```python
from build123d import *

# Parameters (mm, degrees)
SKETCH_1_W          = 47
SKETCH_1_H          = 47
EXTRUDE_1_DEPTH     = 17
SKETCH_2_R          = 2.1
CUT_EXTRUDE_1_DEPTH = 69.607579756
SKETCH_3_W          = 34.6
SKETCH_3_H          = 34.6
CUT_EXTRUDE_2_DEPTH = 14.25
FILLET_1_R          = 2
FILLET_2_R          = 1.5
CHAMFER_1_SIZE      = 1.5
FILLET_3_R          = 1.5


with BuildPart() as part:
    # Эскиз1 → Бобышка-Вытянуть1 (new body)
    with BuildSketch(Plane(origin=(0, 0, 0), x_dir=(1, 0, 0), z_dir=(0, 1, 0))):
        with Locations((-23.5, 23.5)):
            Rectangle(SKETCH_1_W, SKETCH_1_H)
    extrude(amount=EXTRUDE_1_DEPTH)

    # Эскиз2 → Вырез-Вытянуть1 (cut, through all)
    with BuildSketch(Plane.XZ):
        with Locations(Location((-43.5, -3.5, 0), (0, 0, 270))):
            Circle(SKETCH_2_R)
        with Locations(Location((-3.5, -3.5, 0), (0, 0, 90))):
            Circle(SKETCH_2_R)
        with Locations(Location((-3.5, -43.5, 0), (0, 0, 270))):
            Circle(SKETCH_2_R)
        with Locations(Location((-43.5, -43.5, 0), (0, 0, 90))):
            Circle(SKETCH_2_R)
    extrude(amount=-CUT_EXTRUDE_1_DEPTH, mode=Mode.SUBTRACT)

    # Эскиз3 → Вырез-Вытянуть2 (cut)
    with BuildSketch(Plane.XZ):
        with Locations((-23.5, -23.5)):
            Rectangle(SKETCH_3_W, SKETCH_3_H)
    extrude(amount=-CUT_EXTRUDE_2_DEPTH, mode=Mode.SUBTRACT)

    # Скругление1
    fillet_1_edges = [part.edges().sort_by_distance(p)[0] for p in [
        (0, 8.5, 0),
        (-47, 8.5, 0),
        (-47, 8.5, -47),
        (0, 8.5, -47),
    ]]
    fillet(fillet_1_edges, radius=FILLET_1_R)

    # Скругление2
    fillet_2_edges = [part.edges().sort_by_distance(p)[0] for p in [
        (-40.8, 14.25, -23.5),
        (-23.5, 14.25, -6.2),
        (-6.2, 14.25, -23.5),
        (-23.5, 14.25, -40.8),
    ]]
    fillet(fillet_2_edges, radius=FILLET_2_R)

    # Фаска1
    # the kernel refuses this chamfer: 1.5 mm, written as the material it takes off along each edge
    with BuildSketch(Plane(origin=(-43.5, 17, -43.5), x_dir=(0, 0, 1), z_dir=(1, 0, 0))) as chamfer_1_piece_1:
        Polygon((2.1, CHAMFER_1_SIZE), (2.1 + CHAMFER_1_SIZE, 0), (2.1, 0), align=None)
    revolve(axis=Axis((-43.5, 17, -43.5), (0, -1, 0)), mode=Mode.SUBTRACT)
    with BuildSketch(Plane(origin=(-3.5, 17, -43.5), x_dir=(0, 0, -1), z_dir=(-1, 0, 0))) as chamfer_1_piece_2:
        Polygon((2.1, CHAMFER_1_SIZE), (2.1 + CHAMFER_1_SIZE, 0), (2.1, 0), align=None)
    revolve(axis=Axis((-3.5, 17, -43.5), (0, -1, 0)), mode=Mode.SUBTRACT)
    with BuildSketch(Plane(origin=(-3.5, 17, -3.5), x_dir=(0, 0, 1), z_dir=(1, 0, 0))) as chamfer_1_piece_3:
        Polygon((2.1, CHAMFER_1_SIZE), (2.1 + CHAMFER_1_SIZE, 0), (2.1, 0), align=None)
    revolve(axis=Axis((-3.5, 17, -3.5), (0, -1, 0)), mode=Mode.SUBTRACT)
    with BuildSketch(Plane(origin=(-43.5, 17, -3.5), x_dir=(0, 0, -1), z_dir=(-1, 0, 0))) as chamfer_1_piece_4:
        Polygon((2.1, CHAMFER_1_SIZE), (2.1 + CHAMFER_1_SIZE, 0), (2.1, 0), align=None)
    revolve(axis=Axis((-43.5, 17, -3.5), (0, -1, 0)), mode=Mode.SUBTRACT)

    # Скругление3
    # the kernel refuses this fillet: 1.5 mm, written as the material it adds along each edge
    with BuildSketch(Plane(origin=(-39.3, 12.75, -39.3), x_dir=(0, 0, -1), z_dir=(-1, 0, 0))) as fillet_3_piece_1_section:
        Polygon((0, 0), (FILLET_3_R, 0), (FILLET_3_R, -FILLET_3_R), (0, -FILLET_3_R), align=None)
    fillet_3_piece_1 = extrude(amount=FILLET_3_R, mode=Mode.PRIVATE)
    fillet_3_piece_1 = fillet_3_piece_1 - Plane(origin=(-39.3, 12.75, -39.3), x_dir=(0, -0.7071067811865475, 0.7071067811865475), z_dir=(-1, 0, 0)) * Sphere(FILLET_3_R, mode=Mode.PRIVATE)
    add(fillet_3_piece_1)
    with BuildSketch(Plane(origin=(-39.3, 12.75, -7.7), x_dir=(0, 0, 1), z_dir=(-1, 0, 0))) as fillet_3_piece_2_section:
        Polygon((0, 0), (FILLET_3_R, 0), (FILLET_3_R, FILLET_3_R), (0, FILLET_3_R), align=None)
    fillet_3_piece_2 = extrude(amount=FILLET_3_R, mode=Mode.PRIVATE)
    fillet_3_piece_2 = fillet_3_piece_2 - Plane(origin=(-39.3, 12.75, -7.7), x_dir=(0, -0.7071067811865475, -0.7071067811865475), z_dir=(-1, 0, 0)) * Sphere(FILLET_3_R, mode=Mode.PRIVATE)
    add(fillet_3_piece_2)
    with BuildSketch(Plane(origin=(-7.7, 12.75, -39.3), x_dir=(1, 0, 0), z_dir=(0, 0, -1))) as fillet_3_piece_3_section:
        Polygon((0, 0), (FILLET_3_R, 0), (FILLET_3_R, -FILLET_3_R), (0, -FILLET_3_R), align=None)
    fillet_3_piece_3 = extrude(amount=FILLET_3_R, mode=Mode.PRIVATE)
    fillet_3_piece_3 = fillet_3_piece_3 - Plane(origin=(-7.7, 12.75, -39.3), x_dir=(-0.7071067811865475, -0.7071067811865475, 0), z_dir=(0, 0, -1)) * Sphere(FILLET_3_R, mode=Mode.PRIVATE)
    add(fillet_3_piece_3)
    with BuildSketch(Plane(origin=(-7.7, 12.75, -7.7), x_dir=(1, 0, 0), z_dir=(0, 0, 1))) as fillet_3_piece_4_section:
        Polygon((0, 0), (FILLET_3_R, 0), (FILLET_3_R, FILLET_3_R), (0, FILLET_3_R), align=None)
    fillet_3_piece_4 = extrude(amount=FILLET_3_R, mode=Mode.PRIVATE)
    fillet_3_piece_4 = fillet_3_piece_4 - Plane(origin=(-7.7, 12.75, -7.7), x_dir=(-0.7071067811865475, -0.7071067811865475, 0), z_dir=(0, 0, 1)) * Sphere(FILLET_3_R, mode=Mode.PRIVATE)
    add(fillet_3_piece_4)
    with BuildSketch(Plane(origin=(-6.2, 0, -6.2), x_dir=(-1, 0, 0), z_dir=(0, 1, 0)), Plane(origin=(-40.8, 0, -6.2), x_dir=(0, 0, -1), z_dir=(0, 1, 0))) as fillet_3_piece_5:
        with BuildLine():
            CenterArc((FILLET_3_R, -FILLET_3_R), FILLET_3_R, 90, 90)
            Line((0, -FILLET_3_R), (0, 0))
            Line((0, 0), (FILLET_3_R, 0))
        make_face()
    extrude(amount=12.75)
    with BuildSketch(Plane(origin=(-6.2, 0, -40.8), x_dir=(-1, 0, 0), z_dir=(0, 1, 0)), Plane(origin=(-40.8, 0, -40.8), x_dir=(0, 0, 1), z_dir=(0, 1, 0))) as fillet_3_piece_6:
        with BuildLine():
            CenterArc((FILLET_3_R, FILLET_3_R), FILLET_3_R, 180, 90)
            Line((0, FILLET_3_R), (0, 0))
            Line((0, 0), (FILLET_3_R, 0))
        make_face()
    extrude(amount=12.75)


solid = part.part
```
For this review, take the finished solid that the model builds, in its own axes (mm). A direction names the side the tool comes from. Coordinates: 2 decimals unless noted, no trailing zeros. Write each loop counter-clockwise with the first axis right and the second up, starting at its lowest first coordinate (ties: lowest second). Pieces come first, ordered by that corner, then holes.
(1) For pin 1 Ø6.5 at (x, z) = (-43.5, -43.5) entering from -Y; pin 2 Ø5.5 at (x, z) = (-3.5, -3.5) entering from +Y; pin 3 Ø6.5 at (x, z) = (-3.5, -43.5) entering from +Y; pin 4 Ø5 at (x, z) = (-43.5, -3.5) entering from +Y, all flat-tipped, find the tip position at first contact; note any pin that passes through.
(2) Wall thickness on probe 1 along X at (y, z) = (14.25, -3.5); probe 2 along X at (y, z) = (7.5, -27): over which ranges is each line inside the solid? List them lowest first.
(3) The part is to be moulded in two halves that separate along X. For faces 1 (the face through (-46.3, 17, -46.1)), 2 (the face through (-47, 8, -23)), 3 (the face through (-24, 14.25, -23)), say which applies: +X half, -X half, draft (parallel to the pull), parting line (faces both ways), or undercut.
(4) Tool access review of faces 4 (the face through (-0.6, 8.62, -46.43)), 5 (the face through (-24, 6, -40.8)): name each direction out of +Z, -Z, +X, -X, +Y, -Y from which nothing blocks a thin tool from reaching the whole face with its end or side.
(5) Add section D-D on x = -28.5. Give the boundary of the cut face in (y, z), then the cut area to 3 significant figures.
(6) Add section C-C on z = -43.5. Give the boundary of the cut face in (x, y), then the cut area to 3 significant figures.
(7) Add section B-B on y = 11.75. Give the boundary of the cut face in (x, z), then the cut area to 3 significant figures.
(8) Add section A-A on x = -3.5. Give the boundary of the cut face in (y, z).
Answer sheet:
1. pin 1: stops at y = 0
1. pin 2: stops at y = 16.15
1. pin 3: stops at y = 16.65
1. pin 4: stops at y = 15.9
2. probe 1: x = -47 to -45.6, -41.4 to -5.6, -1.4 to 0
2. probe 2: x = -47 to -40.8, -6.2 to 0
3. face 1: draft
3. face 2: -X half
3. face 3: undercut
4. face 4: -Z, +X, +Y, -Y
4. face 5: -Y
5. outline: (0, -47) - (17, -47) - (17, 0) - (0, 0) - (0, -6.2) - (12.75, -6.2) arc R1.5 cw to (14.25, -7.7) - (14.25, -39.3) arc R1.5 cw to (12.75, -40.8) - (0, -40.8) - close
5. area: 307 mm2
6. outline: (-47, 0) - (-45.6, 0) - (-45.6, 15.5) - (-47, 16.9) - close; (-41.4, 0) - (-5.6, 0) - (-5.6, 15.5) - (-7.1, 17) - (-39.9, 17) - (-41.4, 15.5) - close; (-1.4, 0) - (0, 0) - (0, 16.9) - (-1.4, 15.5) - close
6. area: 652 mm2
7. outline: (-47, -45) arc R2 ccw to (-45, -47) - (-2, -47) arc R2 ccw to (0, -45) - (0, -2) arc R2 ccw to (-2, 0) - (-45, 0) arc R2 ccw to (-47, -2) - close; hole circle Ø4.2 at (-43.5, -43.5); hole circle Ø4.2 at (-43.5, -3.5); hole (-40.8, -39.3) arc R1.5 ccw to (-39.3, -40.8) - (-7.7, -40.8) arc R1.5 ccw to (-6.2, -39.3) - (-6.2, -7.7) arc R1.5 ccw to (-7.7, -6.2) - (-39.3, -6.2) arc R1.5 ccw to (-40.8, -7.7) - close; hole circle Ø4.2 at (-3.5, -43.5); hole circle Ø4.2 at (-3.5, -3.5)
7. area: 955 mm2
8. outline: (0, -47) - (16.9, -47) - (15.5, -45.6) - (0, -45.6) - close; (0, -41.4) - (15.5, -41.4) - (17, -39.9) - (17, -7.1) - (15.5, -5.6) - (0, -5.6) - close; (0, -1.4) - (15.5, -1.4) - (16.9, 0) - (0, 0) - close
